```python
from build123d import *

# Parameters (mm, degrees)
SKETCH1_R           = 15
BOSS_EXTRUDE1_DEPTH = 5
SKETCH3_R           = 1.5
CUT_EXTRUDE2_DEPTH  = 5
SKETCH4_R           = 1.5
CUT_EXTRUDE3_DEPTH  = 5
SKETCH5_R           = 3
CUT_EXTRUDE4_DEPTH  = 10


with BuildPart() as part:
    # Sketch1 → Boss-Extrude1 (new body)
    with BuildSketch(Plane(origin=(0, 0, 0), x_dir=(1, 0, 0), z_dir=(0, 1, 0))):
        Circle(SKETCH1_R)
    extrude(amount=BOSS_EXTRUDE1_DEPTH)

    # Sketch3 → Cut-Extrude2 (cut)
    with BuildSketch(Plane.XZ):
        with Locations((-8.5, 8.5)):
            Circle(SKETCH3_R)
        with Locations((8.485281374, 8.485281374)):
            Circle(SKETCH3_R)
        with Locations((-8.485281374, -8.485281374)):
            Circle(SKETCH3_R)
        with Locations((8.470562748, -8.470562748)):
            Circle(SKETCH3_R)
    extrude(amount=-CUT_EXTRUDE2_DEPTH, mode=Mode.SUBTRACT)

    # Sketch4 → Cut-Extrude3 (cut)
    with BuildSketch(Plane(origin=(0, 5, 0), x_dir=(1, 0, 0), z_dir=(0, 1, 0))):
        with Locations((7, 0)):
            Circle(SKETCH4_R)
        with Locations((0, -7)):
            Circle(SKETCH4_R)
        with Locations((-7, 0)):
            Circle(SKETCH4_R)
        with Locations((0, 7)):
            Circle(SKETCH4_R)
    extrude(amount=-CUT_EXTRUDE3_DEPTH, mode=Mode.SUBTRACT)

    # Sketch5 → Cut-Extrude4 (cut)
    with BuildSketch(Plane(origin=(0, 5, 0), x_dir=(1, 0, 0), z_dir=(0, 1, 0))):
        Circle(SKETCH5_R)
    extrude(amount=-CUT_EXTRUDE4_DEPTH, mode=Mode.SUBTRACT)


solid = part.part
```
Input: part model. Units: mm. Frame: model coordinates. Round coordinates to 2 decimals unless told otherwise and drop trailing zeros. Loops run counter-clockwise (first coordinate to the right, second up) from the corner with the lowest first, then second, coordinate; pieces in that order, holes last. Notation, with made-up numbers: (85, 83) - (103, 83) arc R27 cw to (103, 113) - close; hole circle Ø11 at (-17, -2.5). An arc over 180 degrees is marked (long way). One line per item, written item: value. Start each with the question number.
(1) Section D-D, the plane x = -6. Return loops of the section in (y, z).
(2) Section C-C, the plane y = 1.4. Count the separate pieces of the cut face and the enclosed holes in it, plus the area to 3 significant figures.
(3) Contact query for a flat-ended pin moving along its axis: P1, Ø3.5, axis at x = 0, z = 0, coming from the +Y side. Output: stop coordinate, or through.
(4) Section A-A, the plane x = 0. Return loops of the section in (y, z).
(5) Draft query along X for faces 1 (the cylindrical face through (-0.325, 2.535, 8.464)), 2 (the cylindrical face through (-14.985, 2.465, -0.66)), 3 (the flat face through (0, 5, -4)). Return one class per face: +X half, -X half, draft (parallel to the pull), parting line (faces both ways), or undercut.
(6) Ray query, line 1 (Z direction, x = 0, y = 3.7); line 2 (Z direction, x = -9.5, y = 2.05); line 3 (X direction, y = 1.65, z = -1). Return the intervals inside material, ascending. Write a range as [from, to].
(7) Section B-B, the plane z = 0. Return loops of the section in (x, y).
Results below:
1. outline: (0, -13.75) - (5, -13.75) - (5, -1.12) - (0, -1.12) - close; (0, 1.12) - (5, 1.12) - (5, 13.75) - (0, 13.75) - close
2. separate pieces: 1
2. enclosed holes: 9
2. area: 622 mm^2
3. P1: through
4. outline: (0, -15) - (5, -15) - (5, -8.5) - (0, -8.5) - close; (0, -5.5) - (5, -5.5) - (5, -3) - (0, -3) - close; (0, 3) - (5, 3) - (5, 5.5) - (0, 5.5) - close; (0, 8.5) - (5, 8.5) - (5, 15) - (0, 15) - close
5. face 1: undercut
5. face 2: parting line
5. face 3: draft
6. line 1: [-15, -8.5], [-5.5, -3], [3, 5.5], [8.5, 15]
6. line 2: [-11.61, -9.59], [-7.38, 7.38], [9.62, 11.61]
6. line 3: [-14.97, -8.12], [-5.88, -2.83], [2.83, 5.88], [8.12, 14.97]
7. outline: (-15, 0) - (-8.5, 0) - (-8.5, 5) - (-15, 5) - close; (-5.5, 0) - (-3, 0) - (-3, 5) - (-5.5, 5) - close; (3, 0) - (5.5, 0) - (5.5, 5) - (3, 5) - close; (8.5, 0) - (15, 0) - (15, 5) - (8.5, 5) - close
